Answer from the drawing. Dimensions are ordinates in mm from the lowest x, y and z of the part. Coordinates: 2 decimals unless noted, no trailing zeros. Write each loop counter-clockwise with the first axis right and the second up, starting at its lowest first coordinate (ties: lowest second). Pieces come first, ordered by that corner, then holes.
1) The part is cut by section A-A (y = 0.7). Determine the outline of the cut face in (x, z), then the cut area to 3 significant figures.
2) The part is cut by section B-B (z = 1). Determine the outline of the cut face in (x, y), then the cut area to 3 significant figures.
3) Find the intervals of material crossed by line 1 (X direction, y = 0.1, z = 1.25); line 2 (Z direction, x = 16.25, y = 0.1), in increasing order.
4) The part is cut by section C-C (x = 1.5). Determine the outline of the cut face in (y, z).
5) Each of these flat-tipped pins is pushed along its axis until it touches: pin 1 Ø0.7 at (x, y) = (17.5, 1) entering from +Z; pin 2 Ø1 at (x, z) = (8, 5.5) entering from -Y; pin 3 Ø0.7 at (y, z) = (0.5, 13) entering from +X. Where does it stop, or does it pass through?
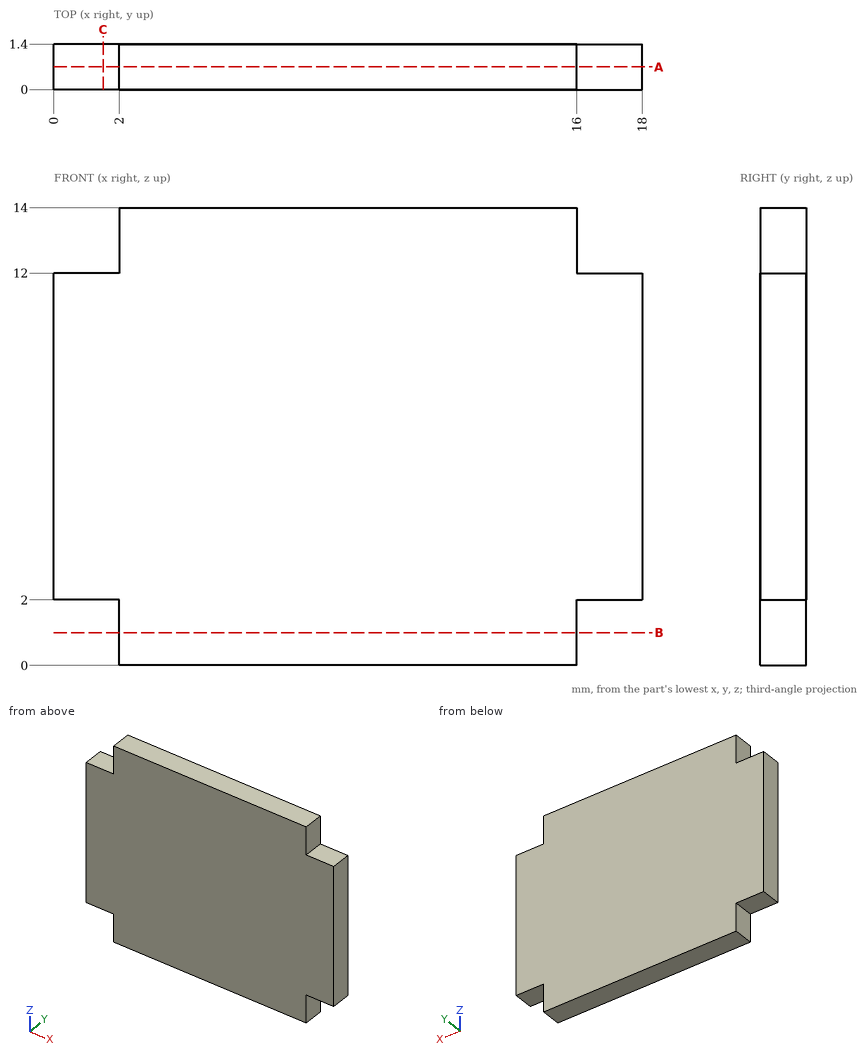
Reported:
1. outline: (0, 2) - (2, 2) - (2, 0) - (16, 0) - (16, 2) - (18, 2) - (18, 12) - (16, 12) - (16, 14) - (2, 14) - (2, 12) - (0, 12) - close
1. area: 236 mm2
2. outline: (2, 0) - (16, 0) - (16, 1.4) - (2, 1.4) - close
2. area: 19.6 mm2
3. line 1: x = 2 to 16
3. line 2: z = 2 to 12
4. outline: (0, 2) - (1.4, 2) - (1.4, 12) - (0, 12) - close
5. pin 1: stops at z = 12
5. pin 2: stops at y = 0
5. pin 3: stops at x = 16
